Drawing for the job (mm, zero at the part's lowest x, y, z). A direction names the side the tool comes from. Coordinates: 2 decimals unless noted, no trailing zeros. Write each loop counter-clockwise with the first axis right and the second up, starting at its lowest first coordinate (ties: lowest second). Pieces come first, ordered by that corner, then holes. Notation, with made-up numbers: (2.5, -1.5) -> (26.5, -1.5) arc R35 cw to (26.5, 35.5) -> close; hole circle Ø4 at (-6.5, 54). An arc over 180 degrees is marked (long way). Write item = value, one per line. Start each with the question number.
Q1. Probe line 1 (Y direction, x = 36.5, z = 5); line 2 (Y direction, x = 7, z = 16); line 3 (Y direction, x = 28, z = 45). List the from-to ranges inside material, lowest first.
Q2. Band-saw the part on C-C, the plane x = 43. List the corners of the cut face in (y, z).
Q3. Band-saw the part on D-D, the plane z = 5. List the corners of the cut face in (x, y), plus the area to 3 significant figures.
Q4. Pin check, flat tips, straight feed: P1, Ø11.5, axis at x = 43, z = 31.5, coming from the -Y side; P2, Ø10.5, axis at x = 41, y = 12, coming from the +Z side; P3, Ø1.5, axis at x = 21.5, y = 29, coming from the +Z side. Stop position of each tip, or through.
Q5. Band-saw the part on B-B, the plane y = 18. List the corners of the cut face in (x, z).
Q6. Tool access for the marked faces 5, 6, 7, 8 and 9: list every direction of +Z, -Z, +X, -X, +Y, -Y with a clear straight run to the whole face (end or side of a thin tool).
Q7. Band-saw the part on A-A, the plane z = 31. List the corners of the cut face in (x, y), plus the area to 3 significant figures.
Q8. Pull direction X, two halves, no side cores. Call the marked faces 1, 2, 3 and 4: released by +X, released by -X, zero draft, split by the parting line, or undercut.
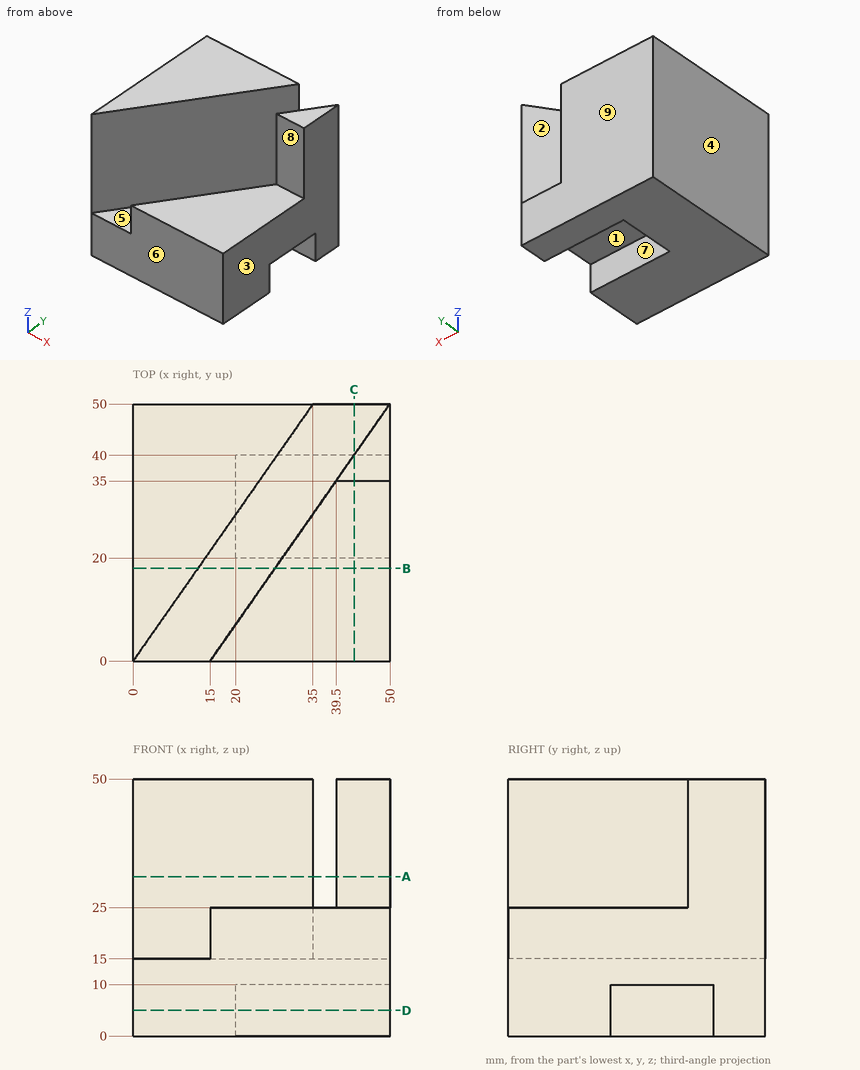
Ans:
q1.line_1 = 0 to 20, 40 to 50
q1.line_2 = 10 to 50
q1.line_3 = 40 to 50
q2.outline = (0, 0) -> (20, 0) -> (20, 10) -> (40, 10) -> (40, 0) -> (50, 0) -> (50, 15) -> (40, 15) -> (40, 50) -> (35, 50) -> (35, 25) -> (0, 25) -> close
q3.outline = (0, 0) -> (50, 0) -> (50, 20) -> (20, 20) -> (20, 40) -> (50, 40) -> (50, 50) -> (0, 50) -> close
q3.area = 1,900 mm2
q4.P1 = 35
q4.P2 = 25
q4.P3 = 15
q5.outline = (0, 0) -> (50, 0) -> (50, 25) -> (27.6, 25) -> (27.6, 15) -> (12.6, 15) -> (12.6, 50) -> (0, 50) -> close
q6.face_5 = +Z
q6.face_6 = +Z, -Z, +X, -X, -Y
q6.face_7 = -Z, +X
q6.face_8 = +Z, +X, -Y
q6.face_9 = +Z, -Z, +X, -X, +Y
q7.outline = (0, 0) -> (35, 50) -> (0, 50) -> close; (39.5, 35) -> (50, 35) -> (50, 50) -> close
q7.area = 954 mm2
q8.face_1 = zero draft
q8.face_2 = undercut
q8.face_3 = released by +X
q8.face_4 = released by -X
